from build123d import *

# Parameters (mm, degrees)
SKETCH_1_W            = 140
SKETCH_1_H            = 140
EXTRUDE_140X140_DEPTH = 10
EXTRUDE_START         = 10
SKETCH_2_W            = 39.6
SKETCH_2_H            = 39.6
SKETCH_2_W_2          = 30
SKETCH_2_H_2          = 30
EXTRUDE_39P6_DEPTH    = 8
M5_M4_DEPTH           = 101.618089825
M5_M4_DEPTH_BACK      = 101.618089825
SKETCH_3_R            = 2.75
SKETCH_3_R_2          = 2.25


with BuildPart() as part:
    # 草图1 → 锚固底板140x140 (new body)
    with BuildSketch(Plane.XY):
        Rectangle(SKETCH_1_W, SKETCH_1_H)
    extrude(amount=EXTRUDE_140X140_DEPTH)

    # 草图2 → 立柱定位凸台39p6 (add)
    with BuildSketch(Plane.XY.offset(EXTRUDE_START)):
        Rectangle(SKETCH_2_W, SKETCH_2_H)
        Rectangle(SKETCH_2_W_2, SKETCH_2_H_2, mode=Mode.SUBTRACT)
    extrude(amount=EXTRUDE_39P6_DEPTH)

    # 草图3 → 桌面M5与立柱M4通孔 (cut, two sides: drawn at the far end of the back side and taken through both)
    with BuildSketch(Plane.XY.offset(-M5_M4_DEPTH_BACK)):
        with Locations((-55, -55)):
            Circle(SKETCH_3_R)
        with Locations((-55, 55)):
            Circle(SKETCH_3_R)
        with Locations((55, -55)):
            Circle(SKETCH_3_R)
        with Locations((55, 55)):
            Circle(SKETCH_3_R)
        with Locations((-32, -32)):
            Circle(SKETCH_3_R_2)
        with Locations((-32, 32)):
            Circle(SKETCH_3_R_2)
        with Locations((32, -32)):
            Circle(SKETCH_3_R_2)
        with Locations((32, 32)):
            Circle(SKETCH_3_R_2)
    extrude(amount=M5_M4_DEPTH + M5_M4_DEPTH_BACK, mode=Mode.SUBTRACT)


solid = part.part
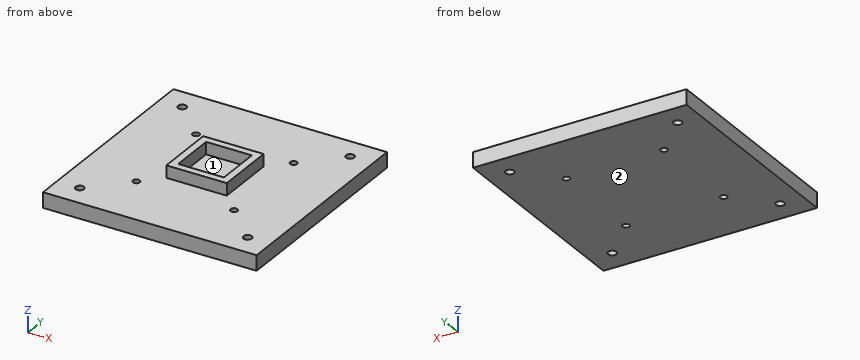
Design review of the part built by this model. Coordinates are the model's own, in mm. Face numbers are marked on the shaded views. Give positions to 0.01 mm unless a question says otherwise; leave off trailing zeros. Write each loop counter-clockwise with the first axis right and the second up, starting at its lowest first coordinate (ties: lowest second). Pieces come first, ordered by that corner, then holes. Notation, with made-up numbers: M 75.25,1 L 130.25,1 A8 cw 130.25,14 Z; hole C 2,10 d7. An arc over 180 degrees is marked long. Answer as a JSON object with one key per item and string values. Group by question number.
1) We need section A-A (x = 55). Give the boundary of the cut face in (y, z).
2) We need section D-D (y = -11). Give the boundary of the cut face in (x, z).
3) We need section B-B (y = 32). Give the boundary of the cut face in (x, z), and give its area (3 significant figures).
4) Mouldability with a two-part tool opening along X and no side actions: class the marked faces 1 and 2 as released by +X, released by -X, zero draft, split by the parting line, or undercut.
5) We need section C-C (z = 14.5). Give the boundary of the cut face in (x, y).
6) Clearance check with flat-ended pins moving along their axes: pin 1 Ø2.5 at (x, z) = (0.5, 13) entering from +Y; pin 2 Ø4 at (x, y) = (22, -47) entering from +Z; pin 3 Ø4.5 at (x, y) = (-55, -55) entering from +Z; pin 4 Ø2.5 at (x, z) = (-4.5, 15.5) entering from -Y. State where each tip first meets the part, or that it passes through.
7) For line 1 along Y through (x, z) = (32, 3.25); line 2 along Y through (x, z) = (-55, 2.75), list the stretches that pass through material, from the lowest coordinate up.
Answer key:
{
 "1": {"outline": "M -70,0 L -57.75,0 L -57.75,10 L -70,10 Z; M -52.25,0 L 52.25,0 L 52.25,10 L -52.25,10 Z; M 57.75,0 L 70,0 L 70,10 L 57.75,10 Z"},
 "2": {"outline": "M -70,0 L 70,0 L 70,10 L 19.8,10 L 19.8,18 L 15,18 L 15,10 L -15,10 L -15,18 L -19.8,18 L -19.8,10 L -70,10 Z"},
 "3": {"outline": "M -70,0 L -34.25,0 L -34.25,10 L -70,10 Z; M -29.75,0 L 29.75,0 L 29.75,10 L -29.75,10 Z; M 34.25,0 L 70,0 L 70,10 L 34.25,10 Z", "area": "1,310 mm²"},
 "4": {"face 1": "undercut", "face 2": "zero draft"},
 "5": {"outline": "M -19.8,-19.8 L 19.8,-19.8 L 19.8,19.8 L -19.8,19.8 Z; hole M -15,-15 L 15,-15 L 15,15 L -15,15 Z"},
 "6": {"pin 1": "stops at y = 19.8", "pin 2": "stops at z = 10", "pin 3": "passes through", "pin 4": "stops at y = -19.8"},
 "7": {"line 1": "y = -70 to -34.25, -29.75 to 29.75, 34.25 to 70", "line 2": "y = -70 to -57.75, -52.25 to 52.25, 57.75 to 70"}
}
